Source: CAD feature listing. Evaluate the final solid. Frame: model axes, mm. Face numbers are marked on the shaded views. A direction names the side the tool comes from. Give positions to 0.01 mm unless a question says otherwise; leave off trailing zeros. Loops run counter-clockwise (first coordinate to the right, second up) from the corner with the lowest first, then second, coordinate; pieces in that order, holes last. Notation, with made-up numbers: (84, 47.25) -> (136, 47.25) arc R31 cw to (136, 86.25) -> close; hole circle Ø5 at (23.5, 53). An arc over 180 degrees is marked (long way). Put each result on its own line as item: value.
```python
from build123d import *

# Parameters (mm, degrees)
F1_DEPTH = 5.08
F2_R     = 1.397
F3_DEPTH = 25.4


with BuildPart() as f1:
    # F0 (on Front) → F1 (new body)
    with BuildSketch(Plane.XZ):
        Polygon((-15.834635, 13.97), (-18.374635, 13.97), (-18.374635, 0), (-12.024635, 0), (-12.024635, 3.81), (-15.834635, 3.81), align=None)
        Polygon((-12.024635, 3.81), (-12.024635, 0), (-5.674635, 0), (-5.674635, 13.97), (-8.214635, 13.97), (-8.214635, 3.81), align=None)
    extrude(amount=F1_DEPTH)

    # F2 (on face) → F3 (cut)
    with BuildSketch(Plane.YZ.offset(-5.674635)):
        with Locations((-2.54, 0)):
            Circle(F2_R)
    extrude(amount=-F3_DEPTH, mode=Mode.SUBTRACT)


solid = f1.part
```
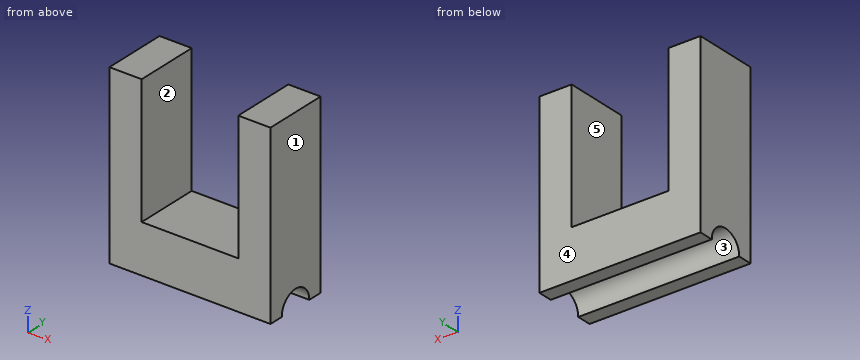
(1) First-contact query: P1, Ø2.5, axis at x = -13.5, y = -3.5, coming from the +Z side. Flat tip, straight axial feed; report the tip coordinate or a pass-through.
Calculated:
P1: stops at z = 3.81
(2) Draft query along X for the marked faces 1, 2 and 3. Return one class per face: released by +X, released by -X, zero draft, split by the parting line, or undercut.
Calculated:
face 1: released by +X
face 2: undercut
face 3: zero draft
(3) Section D-D on y = -2.54. Return loops of the section in (x, z).
Calculated:
outline: (-18.37, 1.4) -> (-5.67, 1.4) -> (-5.67, 13.97) -> (-8.21, 13.97) -> (-8.21, 3.81) -> (-15.83, 3.81) -> (-15.83, 13.97) -> (-18.37, 13.97) -> close
(4) Section C-C on x = -13.25. Return loops of the section in (y, z), then the cut area to 3 significant figures.
Calculated:
outline: (-5.08, 0) -> (-3.94, 0) arc R1.4 cw to (-1.14, 0) -> (0, 0) -> (0, 3.81) -> (-5.08, 3.81) -> close
area: 16.3 mm²
(5) Section B-B on y = -0.4. Return loops of the section in (x, z), then the cut area to 4 significant figures.
Calculated:
outline: (-18.37, 0) -> (-5.67, 0) -> (-5.67, 13.97) -> (-8.21, 13.97) -> (-8.21, 3.81) -> (-15.83, 3.81) -> (-15.83, 13.97) -> (-18.37, 13.97) -> close
area: 100.0 mm²
(6) Line query: probe 1 along X at (y, z) = (-0.85, 9); probe 2 along Z at (x, y) = (-11, -4.5); probe 3 along Z at (x, y) = (-11, -2.6). Output: solid intervals per line, ascending. Write a range as from..to.
Calculated:
probe 1: x = -18.37..-15.83, -8.21..-5.67
probe 2: z = 0..3.81
probe 3: z = 1.4..3.81
(7) Reachability of the marked faces 4 and 5 from +Z, -Z, +X, -X, +Y, -Y: full face, straight path, thin tool, end or side. Return the list, or none.
Calculated:
face 4: +Z, -Z, +X, -X, +Y
face 5: +Z, +Y, -Y
(8) Section A-A on z = 8. Return loops of the section in (x, y), then the cut area to 3 significant figures.
Calculated:
outline: (-18.37, -5.08) -> (-15.83, -5.08) -> (-15.83, 0) -> (-18.37, 0) -> close; (-8.21, -5.08) -> (-5.67, -5.08) -> (-5.67, 0) -> (-8.21, 0) -> close
area: 25.8 mm²
